Part model, mm, in its own coordinate system. Face numbers are marked on the shaded views. A direction names the side the tool comes from. Coordinates: 2 decimals unless noted, no trailing zeros. Loops run counter-clockwise (first coordinate to the right, second up) from the corner with the lowest first, then second, coordinate; pieces in that order, holes last. Notation, with made-up numbers: (52.25, 11.5) - (90.25, 11.5) arc R12 cw to (90.25, 34.5) - close; hole circle Ø4 at (20.25, 82.25). An arc over 180 degrees is marked (long way). Use a Markdown table: item, result. Add a question column.
1. Band-saw the part on D-D, the plane y = -106. Give the cut face in (x, z).
2. Band-saw the part on B-B, the plane z = 17. Give the cut face in (x, y).
3. Drop flat-ended pins along their axis: pin 1 (10 mm diameter, centred on y = -97.5, z = 118, fed in from +X); pin 2 (1.5 mm diameter, centred on x = 52, y = -16.5, fed in from +Z); pin 3 (5 mm diameter, centred on y = -90, z = 16, fed in from +X). Give the stop position or say it passes through.
4. Band-saw the part on C-C, the plane x = 142. Give the cut face in (y, z).
5. Band-saw the part on A-A, the plane y = -7.5. Give the cut face in (x, z), plus the area to 3 significant figures.
6. 3-axis set-ups, long thin cutter, end or side, ignore diameter. For the marked faces 1 and 2: which of +Z, -Z, +X, -X, +Y, -Y reach the whole face in a straight line?
7. Pull direction Y, two halves, no side cores. Call the marked faces 3, 4, 5 and 6: pulls with the +Y half, pulls with the -Y half, needs draft (parallel to the pull), parting line crosses it, or undercut.
8. Wall check: probe 1 along Y at (x, z) = (75, 21.5); probe 2 along Y at (x, z) = (107, 56.5); probe 3 along X at (y, z) = (50, 174). Give the ranges that are in metal, low to high. Write a range as [from, to].
from build123d import *

# Parameters (mm, degrees)
F1_DEPTH = 127
F3_DEPTH = 38.1
F4_DEPTH = 25.4


# Not quite as in the source:
# - a pattern or mirror of a feature is missing from the dataset's text; its kind, count and spacing are read off the source's solid


with BuildPart() as f1:
    # F0 (on Front) → F1 (new body, symmetric)
    with BuildSketch(Plane.XZ):
        Polygon((0, 88.9), (0, 186.69), (-38.1, 215.9), (-38.1, -38.1), (215.9, -38.1), (215.9, 0), (152.4, 0), (0, 0), align=None)
    extrude(amount=F1_DEPTH, both=True)

    # F2 (on face) → F3 (join)
    with BuildSketch(Plane.XZ.offset(127)):
        Polygon((215.9, 0), (0, 114.3), (0, 0), align=None)
    f3 = extrude(amount=-F3_DEPTH)

    # F3_copies: F3 across plane
    add(f3.mirror(Plane.ZX))

    # F0 (on Front) → F4 (join, symmetric)
    with BuildSketch(Plane.XZ):
        Polygon((0, 88.9), (0, 186.69), (-38.1, 215.9), (-38.1, -38.1), (215.9, -38.1), (215.9, 0), (152.4, 0), (0, 0), align=None)
        Polygon((50.8, 88.9), (0, 88.9), (0, 0), (152.4, 0), align=None)
    extrude(amount=F4_DEPTH, both=True)


solid = f1.part
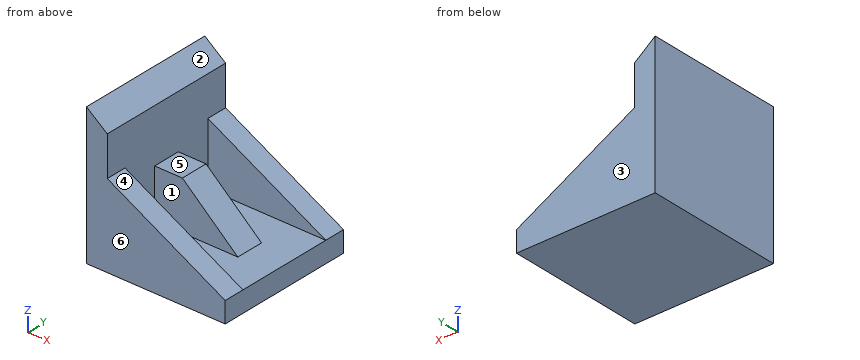
Geometry check:
| question | item | result |
|---|---|---|
| 1 | outline | (-38.1, -38.1) - (215.9, -38.1) - (215.9, 0) - (0, 114.3) - (0, 186.69) - (-38.1, 215.9) - close |
| 2 | outline | (-38.1, -127) - (183.79, -127) - (183.79, -88.9) - (0, -88.9) - (0, -25.4) - (132.97, -25.4) - (132.97, 25.4) - (0, 25.4) - (0, 88.9) - (183.79, 88.9) - (183.79, 127) - (-38.1, 127) - close |
| 3 | pin 1 | stops at x = 2.46 |
| 3 | pin 2 | stops at z = 88.51 |
| 3 | pin 3 | stops at x = 190.4 |
| 4 | outline | (-127, -38.1) - (127, -38.1) - (127, 39.12) - (88.9, 39.12) - (88.9, 0) - (25.4, 0) - (25.4, 9.1) - (-25.4, 9.1) - (-25.4, 0) - (-88.9, 0) - (-88.9, 39.12) - (-127, 39.12) - close |
| 5 | outline | (-38.1, -38.1) - (215.9, -38.1) - (215.9, 0) - (152.4, 0) - (50.8, 88.9) - (0, 88.9) - (0, 186.69) - (-38.1, 215.9) - close |
| 5 | area | 26,400 mm^2 |
| 6 | face 1 | +Z, +X |
| 6 | face 2 | +Z, +X, +Y, -Y |
| 7 | face 3 | pulls with the +Y half |
| 7 | face 4 | needs draft |
| 7 | face 5 | undercut |
| 7 | face 6 | pulls with the -Y half |
| 8 | probe 1 | y = [-127, -88.9], [-25.4, 25.4], [88.9, 127] |
| 8 | probe 2 | y = [-127, -88.9], [88.9, 127] |
| 8 | probe 3 | x = [-38.1, 0] |
